For this review, take the finished solid that the model builds, in its own axes (mm). A direction names the side the tool comes from. Round coordinates to 2 decimals unless told otherwise and drop trailing zeros. Write each loop counter-clockwise with the first axis right and the second up, starting at its lowest first coordinate (ties: lowest second). Pieces come first, ordered by that corner, then holes. Notation, with made-up numbers: M -9,-23.5 L 36,-23.5 A14 ccw 36,-18.5 Z; hole C -25,53.5 d4. An arc over 180 degrees is marked long. One line per question, with ' | ' between items.
Autodesk Inventor part; units mm, degrees
ref_plane "bolt_to_nut_XY" through (8, 0, 0) normal (1, 0, 0) x (0, 0, -1)
ref_plane "bolt_to_nut_YZ" through (8, 0, 0) normal (0, 0, -1) x (0, 1, 0)
ref_plane "bolt_to_nut_ZX" through (8, 0, 0) normal (0, 1, 0) x (1, 0, 0)
sketch "Sketch_1" plane through (0, 0, 0) normal (0, 0, 1) x (1, 0, 0)
  line L0 (8, 0) -> (-2.5, 0)
  line L1 (-2.5, 0) -> (-2.5, 2)
  line L2 (-2.5, 2) -> (-2.25, 2.25)
  line L3 (-2.25, 2.25) -> (0, 2.25)
  line L4 (0, 2.25) -> (0, 1.25)
  line L5 (0, 1.25) -> (7.724, 1.25)
  line L6 (7.724, 1.25) -> (8, 0.974)
  line L7 (8, 0.974) -> (8, 0)
  line L8 (8, 0) -> (-2.5, 0)
revolve "Revolution1" add sketch "Sketch_1" angle 360 about axis through (8, 0, 0) along (1, 0, 0)
thread "Thread1"
sketch "Sketch2" plane through (-2.5, 0, 0) normal (-1, 0, 0) x (0, 0, 1)
  point P0 (0, 0)
hole "Hole1" at (-2.5, 0, 0) direction (1, 0, 0) diameter 2 depth 1.25 tip angle 150
sketch "Sketch_3" plane through (-2.5, 0, 0) normal (1, 0, 0) x (0, 0, -1)
  line L0 (-1, -0.5774) -> (0, -1.1547)
  line L1 (0, -1.1547) -> (1, -0.5774)
  line L2 (1, -0.5774) -> (1, 0.5774)
  line L3 (1, 0.5774) -> (0, 1.1547)
  line L4 (0, 1.1547) -> (-1, 0.5774)
  line L5 (-1, 0.5774) -> (-1, -0.5774)
extrude "Extrusion1" cut sketch "Sketch_3" along normal blind 1.25
ref_plane "bolt_to_nut_XY" through (8, 0, 0) normal (1, 0, 0) x (0, 0, -1)
ref_plane "bolt_to_nut_YZ" through (8, 0, 0) normal (0, 0, -1) x (0, 1, 0)
ref_plane "bolt_to_nut_ZX" through (8, 0, 0) normal (0, 1, 0) x (1, 0, 0)
ref_plane "screw1_XY" through (0, 0, 0) normal (1, 0, 0) x (0, 0, -1)
ref_plane "screw1_YZ" through (0, 0, 0) normal (0, 0, -1) x (0, 1, 0)
ref_plane "screw1_ZX" through (0, 0, 0) normal (0, 1, 0) x (1, 0, 0)
properties part number "CB2_5-8" material "鋼、炭素鋼"
Item 1: To check wall thickness, follow line 1 along X through (y, z) = (-0.9, 1.55); line 2 along Z through (x, y) = (5, 0); line 3 along Z through (x, y) = (4.5, -0.75). State the ranges of each line that lie inside material, in increasing order. Write a range as from..to.
Results:
line 1: -2.5..0 | line 2: -1.25..1.25 | line 3: -1..1
Item 2: Take a section at A-A (x = 4). Write out the cut boundary in (y, z).
Results:
outline: C 0,0 d2.5
Item 3: Insertion check: pin 1 Ø1 at (x, z) = (6.5, 0) entering from -Y; pin 2 Ø1.5 at (x, z) = (7, 1) entering from +Y. Each pin has a flat end and moves straight along its axis. Give the tip position at first contact, or say it passes through.
Results:
pin 1: y = -1.25 | pin 2: y = 1.22
Item 4: Mouldability with a two-part tool opening along Y and no side actions: class faces 4 (the face through (-1.11, -0.29, 2.23)), 5 (the face through (-1, -0.06, -0.01)), 6 (the face through (0, 1, -1)) as +Y half, -Y half, draft (parallel to the pull), parting line (faces both ways), or undercut.
Results:
face 4: parting line | face 5: undercut | face 6: draft
Item 5: Machinability: for faces 1 (the face through (8, 0, 0)), 2 (the face through (3.92, -0.27, -1.22)), 3 (the face through (-1.88, 0.87, 0.49)), which of the approach directions +Z, -Z, +X, -X, +Y, -Y give a long, thin tool a straight path to every point of the face, cutting with its end or side? Answer none if there is none.
Results:
face 1: +Z, -Z, +X, +Y, -Y | face 2: +X | face 3: -X
